Here's how the part is built. I have some questions about the finished solid (model axes, mm). Give positions to 0.01 mm unless a question says otherwise; leave off trailing zeros. Loops run counter-clockwise (first coordinate to the right, second up) from the corner with the lowest first, then second, coordinate; pieces in that order, holes last. Notation, with made-up numbers: M 55.25,86.25 L 97.25,86.25 A29 cw 97.25,107.25 Z; hole C -3,-11.75 d2. An arc over 180 degrees is marked long. Answer as CSV lines item,"result". Start each with the question number.
Item 1: If I drill on line 1 along Y through (x, z) = (0, 2.5); line 2 along Y through (x, z) = (10.87, 5.25); line 3 along Y through (x, z) = (12, 5.5), over which ranges is the centre line in solid material (lowest first)? Write a range as from..to.
Item 2: I want a section at D-D on y = -20. List the corners of the cut face in (x, z) for me, plus the area to 3 significant figures.
Item 3: If we mould it in two halves opening along X, with no side actions, what happens to faces 1 (the cylindrical face through (-12.465, 56.133, 3.204)), 2 (the cylindrical face through (-0.26, 8.887, 3.204)), 3 (the flat face through (-1, 14, 6.5))? For each: released by +X, released by -X, zero draft, split by the parting line, or undercut.
Item 4: Will these pins go through, and if not, where does the flat tip stop? P1, Ø1, axis at y = -33.5, z = 5, coming from the +X side; P2, Ø1, axis at y = -33, z = 2.5, coming from the -X side; P3, Ø3, axis at y = -31.5, z = 5, coming from the -X side.
Item 5: I want a section at A-A on x = 0. List the corners of the cut face in (y, z) for me, plus the area to 3 significant figures.
Item 6: I want a section at C-C on z = 3. List the corners of the cut face in (x, y) for me.
Autodesk Fusion 360 part; units mm, degrees
sketch "Sketch1" plane through (0, 0, 0) normal (0, 0, 1) x (1, 0, 0)
  circle A0 centre (0, 0) radius 57.5
  circle A1 centre (0, 0) radius 2.5
  line L0 (0, 0) -> (0, 10.87) construction
  circle A2 centre (0, 10.87) radius 2
  circle A3 centre (-10.87, 0) radius 2
  circle A4 centre (0, -10.87) radius 2
  circle A5 centre (10.87, 0) radius 2
  dimension "d1" = 115
  dimension "d2" = 5
  dimension "d3" = 10.87
  dimension "d4" = 4
  dimension "d6" = 360
extrude "Extrude1" add sketch "Sketch1" along normal blind 6.5
Result:
1,line 1,"-57.5..-12.87, -8.87..-2.5, 2.5..8.87, 12.87..57.5"
1,line 2,"-56.46..-2, 2..56.46"
1,line 3,"-56.23..-1.65, 1.65..56.23"
2,outline,"M -53.91,0 L 53.91,0 L 53.91,6.5 L -53.91,6.5 Z"
2,area,"701 mm^2"
3,face 1,"split by the parting line"
3,face 2,"undercut"
3,face 3,"zero draft"
4,P1,"x = 47.09"
4,P2,"x = -47.43"
4,P3,"x = -49.05"
5,outline,"M -57.5,0 L -12.87,0 L -12.87,6.5 L -57.5,6.5 Z; M -8.87,0 L -2.5,0 L -2.5,6.5 L -8.87,6.5 Z; M 2.5,0 L 8.87,0 L 8.87,6.5 L 2.5,6.5 Z; M 12.87,0 L 57.5,0 L 57.5,6.5 L 12.87,6.5 Z"
5,area,"663 mm^2"
6,outline,"C 0,0 d115; hole C -10.87,0 d4; hole C 0,0 d5; hole C 0,-10.87 d4; hole C 0,10.87 d4; hole C 10.87,0 d4"
